CAD build for the part. Positions are in the model's coordinates, mm. Coordinates: 2 decimals unless noted, no trailing zeros. Order: outer loops, then holes, each group sorted by start corner. A loop starts at its lowest first (then second) coordinate and runs counter-clockwise, first axis right, second up. Notation, with made-up numbers: (52, -25.75) -> (93, -25.75) arc R21 ccw to (93, -14.75) -> close; hole circle Ø11 at (-30, 14). An arc over 180 degrees is marked (long way). Use one line per item in the form item = value. Start each with the question number.
from build123d import *

# Parameters (mm, degrees)
F0_W     = 60.5
F0_H     = 41
F1_DEPTH = 1.5
F2_SIZE  = 3
F3_R     = 1.54
F4_DEPTH = 1.5


with BuildPart() as f1:
    # F0 (on Top) → F1 (new body)
    with BuildSketch(Plane.XY):
        with Locations((30.25, 20.5)):
            Rectangle(F0_W, F0_H)
    extrude(amount=F1_DEPTH)

    # F2
    f2_edges = [f1.edges().sort_by_distance(p)[0] for p in [
        (0, 0, 0.75),
    ]]
    chamfer(f2_edges, length=F2_SIZE)

    # F3 (on face) → F4 (cut, through all)
    with BuildSketch(Plane.XY.offset(1.5)):
        with Locations((4, 4)):
            Circle(F3_R)
    extrude(amount=-F4_DEPTH, mode=Mode.SUBTRACT)


solid = f1.part
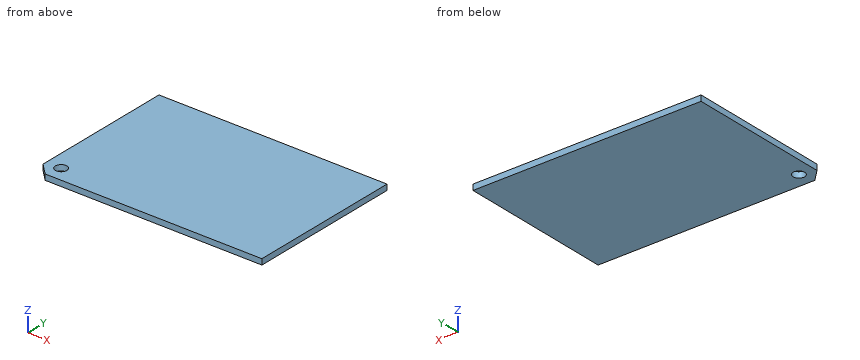
1) Cut at A-A on x = 4. Give the cut face in (y, z).
2) Probe L1, parallel to Y at x = 4, z = 1.1. List the from-to ranges inside material, lowest first.
3) Drop a flat-ended pin along its axis: P1, Ø3, axis at x = 4, y = 4, coming from the +Z side. Give the stop position or say it passes through.
4) Cut at B-B on y = 4. Give the cut face in (x, z), then the cut area to 3 significant figures.
Values follow:
q1.outline = (0, 0) -> (2.46, 0) -> (2.46, 1.5) -> (0, 1.5) -> close; (5.54, 0) -> (41, 0) -> (41, 1.5) -> (5.54, 1.5) -> close
q2.L1 = 0 to 2.46, 5.54 to 41
q3.P1 = through
q4.outline = (0, 0) -> (2.46, 0) -> (2.46, 1.5) -> (0, 1.5) -> close; (5.54, 0) -> (60.5, 0) -> (60.5, 1.5) -> (5.54, 1.5) -> close
q4.area = 86.1 mm^2
